For this review, use the dimensioned drawing (mm, ordinates from the lowest corner) and the shaded views. Coordinates: 2 decimals unless noted, no trailing zeros. Order: outer loops, then holes, each group sorted by start corner. A loop starts at its lowest first (then second) coordinate and runs counter-clockwise, first axis right, second up. Notation, with made-up numbers: M 42.25,47.5 L 101.25,47.5 A14 cw 101.25,53.5 Z; hole C 15,77 d10. An arc over 180 degrees is marked long. Use CSV: the item, a comma, the result in double quotes.
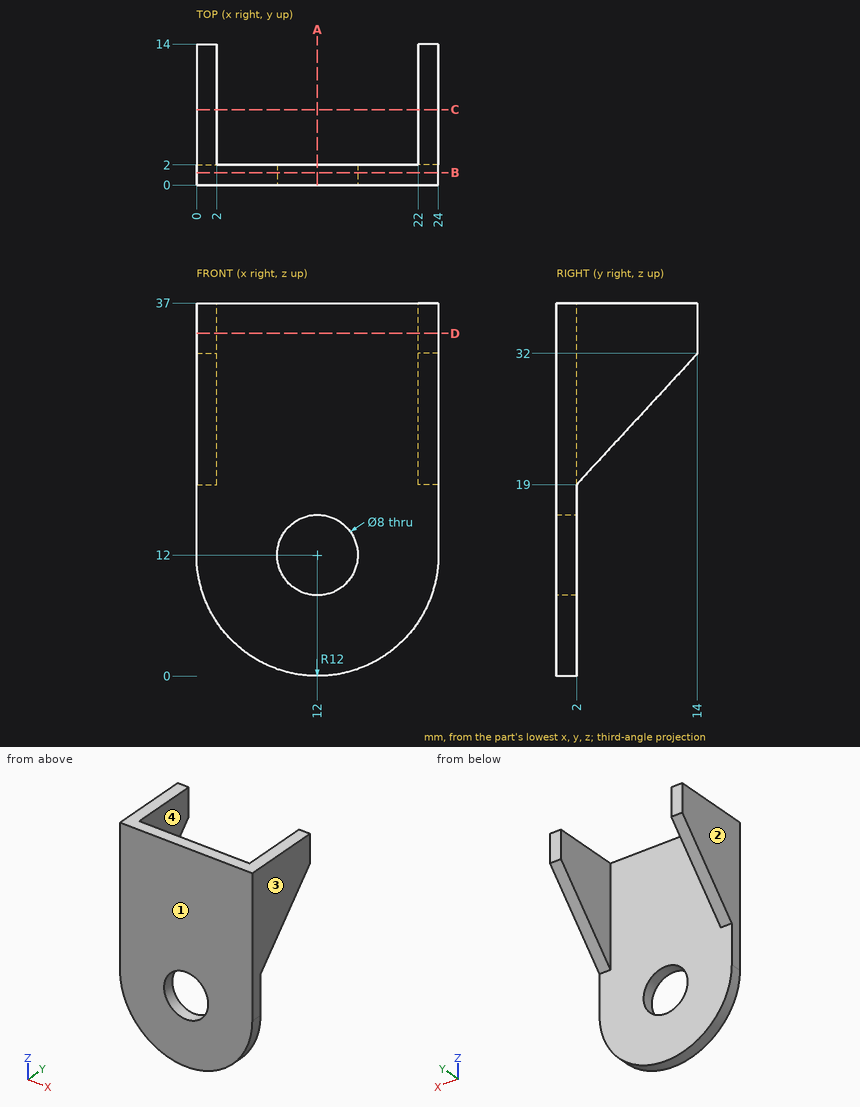
Item 1: To check wall thickness, follow line 1 along X through (y, z) = (0.7, 12); line 2 along X through (y, z) = (4.25, 32.5); line 3 along Y through (x, z) = (15.25, 32.5). State the ranges of each line that lie inside material, in increasing order. Write a range as [from, to].
Solutions:
line 1,"[0, 8], [16, 24]"
line 2,"[0, 2], [22, 24]"
line 3,"[0, 2]"
Item 2: Add section B-B on y = 1.25. State the section outline as (x, z) points.
Solutions:
outline,"M 0,12 A12 ccw 24,12 L 24,37 L 0,37 Z; hole C 12,12 d8"
Item 3: Add section A-A on x = 12. State the section outline as (y, z) points.
Solutions:
outline,"M 0,0 L 2,0 L 2,8 L 0,8 Z; M 0,16 L 2,16 L 2,37 L 0,37 Z"
Item 4: Add section D-D on z = 34. State the section outline as (x, y) points, and give its area (3 significant figures).
Solutions:
outline,"M 0,0 L 24,0 L 24,14 L 22,14 L 22,2 L 2,2 L 2,14 L 0,14 Z"
area,"96.0 mm^2"
Item 5: Clearance check with flat-ended pins moving along their axes: pin 1 Ø12 at (x, z) = (15, 23) entering from +Y; pin 2 Ø8 at (x, y) = (14.5, 7) entering from -Z. State where each tip first meets the part, or that it passes through.
Solutions:
pin 1,"y = 2"
pin 2,"through"
Item 6: Add section C-C on y = 7.5. State the section outline as (x, z) points.
Solutions:
outline,"M 0,24.96 L 2,24.96 L 2,37 L 0,37 Z; M 22,24.96 L 24,24.96 L 24,37 L 22,37 Z"
Item 7: Draft analysis for pull direction X (two halves, no side actions). For the marked faces 1, 2, 3 and 4, state which applies: released by +X, released by -X, zero draft, split by the parting line, or undercut.
Solutions:
face 1,"zero draft"
face 2,"released by -X"
face 3,"released by +X"
face 4,"undercut"
